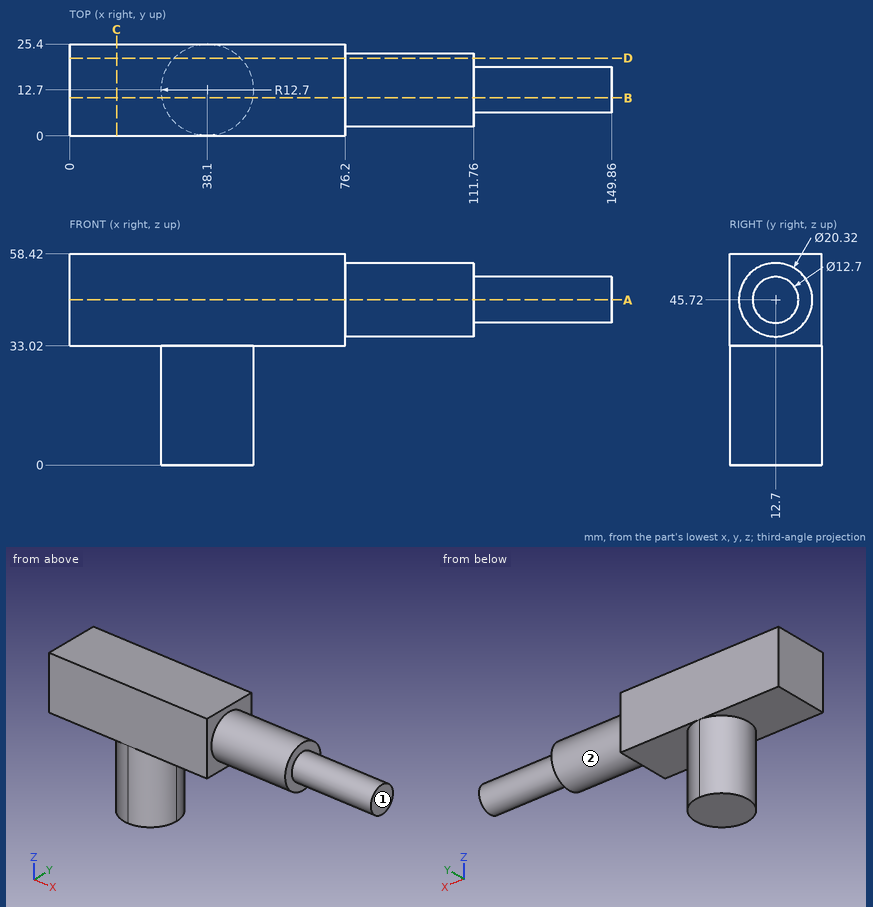
Verification items for this drawing (mm, ordinates from the low corner). A direction names the side the tool comes from. Give positions to 0.01 mm unless a question says otherwise; leave off trailing zeros. Loops run counter-clockwise (first coordinate to the right, second up) from the corner with the lowest first, then second, coordinate; pieces in that order, holes last. Notation, with made-up numbers: M 63.5,-10 L 95.5,-10 A20 cw 95.5,13 Z; hole C 28,-11.5 d11. An arc over 180 degrees is marked long. Write item = value, one per line. Start each with the question number.
1. Section check B-B, the plane y = 10.5. Enter the section's corners in (x, z).
2. Go/stop test with flat-tipped pins: P1, Ø2, axis at x = 89.5, y = 2.5, coming from the -Z side; P2, Ø2, axis at x = 62, y = 21.5, coming from the -Z side; P3, Ø8, axis at x = 109.5, y = 7, coming from the +Z side. Record where each tip stops, or that it passes through.
3. Section check D-D, the plane y = 21.5. Enter the section's corners in (x, z).
4. Tool access check on the marked faces 1 and 2. Record the directions out of +Z, -Z, +X, -X, +Y, -Y that give a thin tool (end or side, any length) a straight path to the whole face; none if there is none.
5. Thickness scan on probe 1 along Z at (x, y) = (11, 19.25); probe 2 along Z at (x, y) = (92, 13); probe 3 along X at (y, z) = (14.5, 35). Record the ranges inside material, lowest first.
6. Section check A-A, the plane z = 45.72. Enter the section's corners in (x, y).
7. Section check C-C, the plane x = 13. Enter the section's corners in (y, z), plus the area to 3 significant figures.
Values follow:
q1.outline = M 0,33.02 L 25.59,33.02 L 25.59,0 L 50.61,0 L 50.61,33.02 L 76.2,33.02 L 76.2,35.8 L 111.76,35.8 L 111.76,39.76 L 149.86,39.76 L 149.86,51.68 L 111.76,51.68 L 111.76,55.64 L 76.2,55.64 L 76.2,58.42 L 0,58.42 Z
q2.P1 = 41.41
q2.P2 = 33.02
q2.P3 = 55.74
q3.outline = M 0,33.02 L 28.94,33.02 L 28.94,0 L 47.26,0 L 47.26,33.02 L 76.2,33.02 L 76.2,40.64 L 111.76,40.64 L 111.76,50.8 L 76.2,50.8 L 76.2,58.42 L 0,58.42 Z
q4.face_1 = +Z, -Z, +X, +Y, -Y
q4.face_2 = +X
q5.probe_1 = 33.02 to 58.42
q5.probe_2 = 35.56 to 55.88
q5.probe_3 = 0 to 76.2
q6.outline = M 0,0 L 76.2,0 L 76.2,2.54 L 111.76,2.54 L 111.76,6.35 L 149.86,6.35 L 149.86,19.05 L 111.76,19.05 L 111.76,22.86 L 76.2,22.86 L 76.2,25.4 L 0,25.4 Z
q7.outline = M 0,33.02 L 25.4,33.02 L 25.4,58.42 L 0,58.42 Z
q7.area = 645 mm^2
